from build123d import *

# Parameters (mm, degrees)
SKETCH1_R           = 76.2
SKETCH1_R_2         = 73.025
BOSS_EXTRUDE1_DEPTH = 76.2
SKETCH3_R           = 76.2
BOSS_EXTRUDE2_DEPTH = 34.417
SKETCH5_R           = 2.1828125
CUT_EXTRUDE2_DEPTH  = 35.417
SKETCH11_R          = 2.1828125
CUT_EXTRUDE11_DEPTH = 35.417
SKETCH12_R          = 3.175
CUT_EXTRUDE12_DEPTH = 35.417


with BuildPart() as part:
    # Sketch1 → Boss-Extrude1 (new body)
    with BuildSketch(Plane.XY):
        Circle(SKETCH1_R)
        Circle(SKETCH1_R_2, mode=Mode.SUBTRACT)
    extrude(amount=BOSS_EXTRUDE1_DEPTH)

    # Sketch3 → Boss-Extrude2 (add)
    with BuildSketch(Plane.XY):
        Circle(SKETCH3_R)
    extrude(amount=BOSS_EXTRUDE2_DEPTH)

    # Sketch5 → Cut-Extrude2 (cut, through all)
    with BuildSketch(Plane.XY.offset(34.417)):
        with Locations((0, 37.81298)):
            Circle(SKETCH5_R)
        with Locations((37.81298, 0)):
            Circle(SKETCH5_R)
        with Locations((-37.81298, 0)):
            Circle(SKETCH5_R)
        with Locations((0, -37.81298)):
            Circle(SKETCH5_R)
    extrude(amount=-CUT_EXTRUDE2_DEPTH, mode=Mode.SUBTRACT)

    # Sketch11 → Cut-Extrude11 (cut, through all)
    with BuildSketch(Plane.XY.offset(34.417)):
        with Locations((-35.921024484, 35.921024484)):
            Circle(SKETCH11_R)
        with Locations((-35.921024484, -35.921024484)):
            Circle(SKETCH11_R)
        with Locations((35.921024484, -35.921024484)):
            Circle(SKETCH11_R)
        with Locations((35.921024484, 35.921024484)):
            Circle(SKETCH11_R)
    extrude(amount=-CUT_EXTRUDE11_DEPTH, mode=Mode.SUBTRACT)

    # Sketch12 → Cut-Extrude12 (cut, through all)
    with BuildSketch(Plane.XY.offset(34.417)):
        Circle(SKETCH12_R)
    extrude(amount=-CUT_EXTRUDE12_DEPTH, mode=Mode.SUBTRACT)


solid = part.part
Work out the finished part from the listing and answer in its coordinate system (mm). A direction names the side the tool comes from. Round coordinates to 2 decimals unless told otherwise and drop trailing zeros. Write each loop counter-clockwise with the first axis right and the second up, starting at its lowest first coordinate (ties: lowest second). Pieces come first, ordered by that corner, then holes. Notation, with made-up numbers: M 86,53.5 L 109,53.5 A19 ccw 109,69.5 Z; hole C 85,34.5 d5. An arc over 180 degrees is marked long. Use a Markdown table: item, result.
1) The part is cut by section A-A on y = 0. Give the vertices of the cut face in (x, z) (3 decimals).
Taken from the geometry:
| item | result |
|---|---|
| outline | M -76.2,0 L -39.996,0 L -39.996,34.417 L -73.025,34.417 L -73.025,76.2 L -76.2,76.2 Z; M -35.63,0 L -3.175,0 L -3.175,34.417 L -35.63,34.417 Z; M 3.175,0 L 35.63,0 L 35.63,34.417 L 3.175,34.417 Z; M 39.996,0 L 76.2,0 L 76.2,76.2 L 73.025,76.2 L 73.025,34.417 L 39.996,34.417 Z |
2) The part is cut by section C-C on z = 20. State how many separate pieces and enclosed holes the cut face has, plus the area to 3 significant figures.
Taken from the geometry:
| item | result |
|---|---|
| separate pieces | 1 |
| enclosed holes | 9 |
| area | 18,100 mm2 |
3) Which of the six approach directions +Z, -Z, +X, -X, +Y, -Y give full straight-line access (tool end or side, diameter ignored) to faces 4 (the face through (69.653, 21.935, 55.016)), 5 (the face through (39, -62, 76.2))?
Taken from the geometry:
| item | result |
|---|---|
| face 4 | +Z |
| face 5 | +Z, +X, -X, +Y, -Y |
4) Determine the mould class of faces 1 (the face through (-0.69, -3.1, 17.45)), 2 (the face through (-60.47, -46.367, 37.567)), 3 (the face through (16, 1, 0)) for opening direction Y: pulls with the +Y half, pulls with the -Y half, needs draft (parallel to the pull), parting line crosses it, or undercut.
Taken from the geometry:
| item | result |
|---|---|
| face 1 | undercut |
| face 2 | parting line crosses it |
| face 3 | needs draft |
5) Consider line 1 (Z direction, x = -4, y = 64.5); line 2 (X direction, y = 11.5, z = 42); line 3 (Y direction, x = 59, z = 42). Determine where each line is inside the solid, lowest interval first. Write a range as [from, to].
Taken from the geometry:
| item | result |
|---|---|
| line 1 | z = [0, 34.42] |
| line 2 | x = [-75.33, -72.11], [72.11, 75.33] |
| line 3 | y = [-48.22, -43.03], [43.03, 48.22] |
6) The part is cut by section D-D on y = 20. Give the vertices of the cut face in (x, z).
Taken from the geometry:
| item | result |
|---|---|
| outline | M -73.53,0 L 73.53,0 L 73.53,76.2 L 70.23,76.2 L 70.23,34.42 L -70.23,34.42 L -70.23,76.2 L -73.53,76.2 Z |
7) Flat-ended cylindrical pins translate along their axes: pin 1 (4 mm diameter, centred on x = 1, y = 54.5, fed in from +Z); pin 2 (4 mm diameter, centred on x = 0, y = 37.81, fed in from +Z); pin 3 (1.5 mm diameter, centred on y = -33.5, z = 16, fed in from -X); pin 4 (8 mm diameter, centred on y = 61, z = 16, fed in from -X). Find the tip coordinate at first contact, or state that the pin passes through.
Taken from the geometry:
| item | result |
|---|---|
| pin 1 | stops at z = 34.42 |
| pin 2 | passes through |
| pin 3 | stops at x = -68.8 |
| pin 4 | stops at x = -50.57 |
